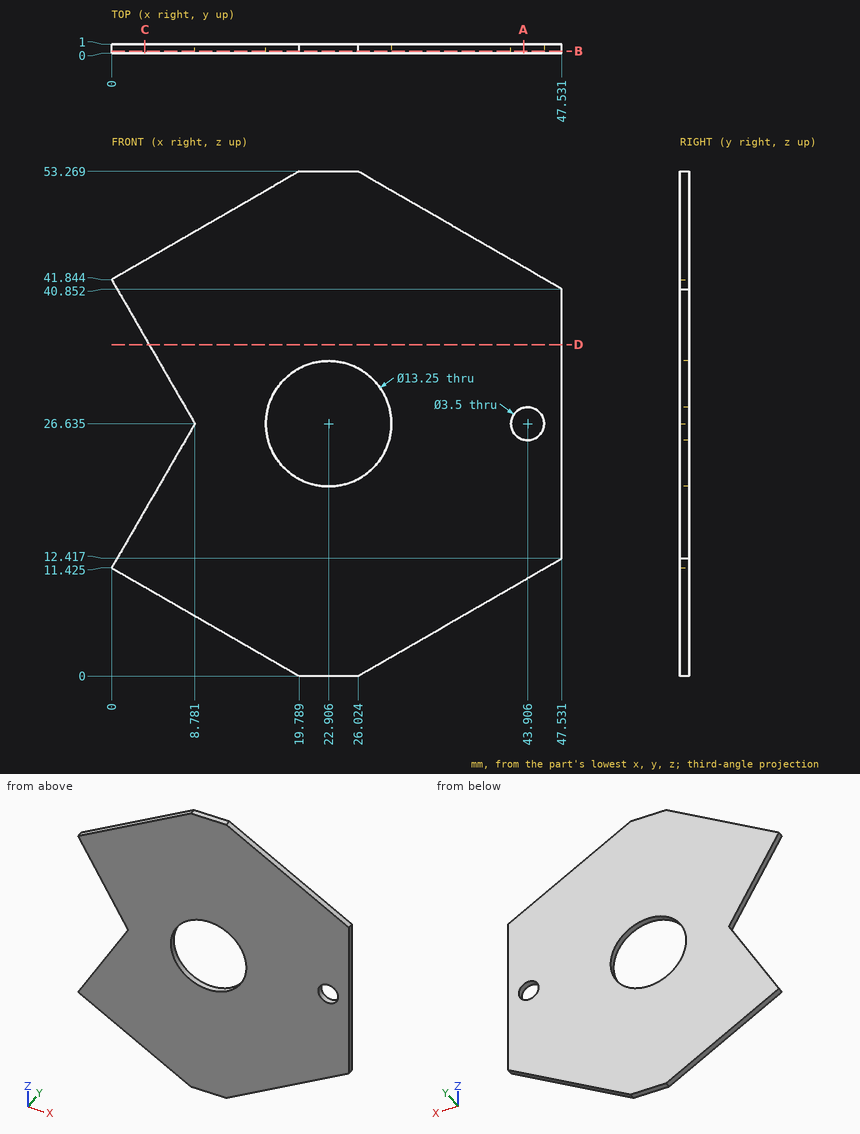
Verification items for this drawing (mm, ordinates from the low corner). Round coordinates to 2 decimals unless told otherwise and drop trailing zeros. Write each loop counter-clockwise with the first axis right and the second up, starting at its lowest first coordinate (ties: lowest second). Pieces come first, ordered by that corner, then holes. Notation, with made-up numbers: (4, 7) - (36, 7) arc R26 cw to (36, 22) - close; hole circle Ø4 at (80, 31). An arc over 180 degrees is marked (long way). One line per item, written item: value.
1. Cross-section at D-D on z = 35. Record the boundary of the cut face in (x, y).
The answers:
outline: (3.95, 0) - (47.53, 0) - (47.53, 1) - (3.95, 1) - close
2. Cross-section at A-A on x = 43.5. Record the boundary of the cut face in (y, z).
The answers:
outline: (0, 10.09) - (1, 10.09) - (1, 24.93) - (0, 24.93) - close; (0, 28.34) - (1, 28.34) - (1, 43.18) - (0, 43.18) - close
3. Depth check by flat-ended pin: pin 1 Ø4 at (x, z) = (43.91, 26.63) entering from +Y. Enter the tip coordinate at first touch or a pass-through.
The answers:
pin 1: stops at y = 1
4. Cross-section at B-B on y = 0.25. Give the number of separate pieces and of enclosed holes in the cut face, and give its area (3 significant figures).
The answers:
separate pieces: 1
enclosed holes: 2
area: 1,760 mm^2
5. Scan lines: L1, parallel to X at y = 0.9, z = 27 (1 decimal); L2, parallel to Z at x = 19.5, y = 0.7 (1 decimal); L3, parallel to Z at x = 23, y = 0.8. Record each from-to range of solid material in increasing order.
The answers:
L1: x = 8.6 to 16.3, 29.5 to 42.2, 45.6 to 47.5
L2: z = 0.2 to 21, 32.3 to 53.1
L3: z = 0 to 20.01, 33.26 to 53.27
6. Cross-section at C-C on x = 3.5. Record the boundary of the cut face in (y, z) (1 decimal).
The answers:
outline: (0, 9.4) - (1, 9.4) - (1, 17.5) - (0, 17.5) - close; (0, 35.8) - (1, 35.8) - (1, 43.9) - (0, 43.9) - close
